The listing builds one solid part. Answer for the finished solid, in the listing's coordinates (mm). Give positions to 0.01 mm unless a question says otherwise; leave off trailing zeros. Order: outer loops, then holes, each group sorted by start corner. A loop starts at its lowest first (then second) coordinate and runs counter-clockwise, first axis right, second up.
Autodesk Inventor part; units mm, degrees
ref_plane "YZ Plane" through (0, 0, 0) normal (1, 0, 0) x (0, 1, 0)
ref_plane "XZ Plane" through (0, 0, 0) normal (0, 1, 0) x (-1, 0, 0)
ref_plane "XY Plane" through (0, 0, 0) normal (0, 0, 1) x (1, 0, 0)
sketch "Sketch1" plane through (0, 0, 0) normal (0, 0, 1) x (1, 0, 0)
  line L0 (0, 0) -> (1300, 0)
  line L1 (1300, 0) -> (1300, 50)
  line L2 (1300, 50) -> (0, 50)
  line L3 (0, 50) -> (0, 0)
  line L4 (0, 50) -> (50, 50)
  line L5 (50, 50) -> (50, 25)
  circle A0 centre (50, 25) radius 10.5
  line L6 (650, 50) -> (650, 17.5)
  circle A1 centre (1288, 40) radius 3
  circle A2 centre (1288, 10) radius 3
  line L7 (1182.5, 14.5) -> (1227.5, 14.5)
  line L8 (1227.5, 14.5) -> (1227.5, 35.5)
  line L9 (1227.5, 35.5) -> (1182.5, 35.5)
  line L10 (1182.5, 35.5) -> (1182.5, 14.5)
  dimension "d0" = 1300
  dimension "d1" = 50
  dimension "d4" = 50
  dimension "d5" = 21
  dimension "d10" = 6
  dimension "d11" = 6
  dimension "d14" = 45
  dimension "d17" = 21
  dimension "d18" = 14.5
  dimension "d19" = 25
  dimension "d20" = 12
  dimension "d21" = 12
  dimension "d22" = 10
extrude "Extrusion4" add sketch "Sketch1" along normal blind 6
equation "\"d18\" = -0.5 * d17 + 0.5 * d1"
properties part number "convyerwall"
1) Find section A-A (z = 2.25). Write down the section's boundary in (x, y).
Geometry says:
outline: (0, 0) - (1300, 0) - (1300, 50) - (0, 50) - close; hole circle Ø21 at (50, 25); hole (1182.5, 14.5) - (1227.5, 14.5) - (1227.5, 35.5) - (1182.5, 35.5) - close; hole circle Ø6 at (1288, 10); hole circle Ø6 at (1288, 40)
2) For a pull along X with two mould halves and no side action, classify faces 1 (the flat face through (641, 25, 6)), 2 (the cylindrical face through (39.51, 24.54, 2.96)) as +X half, -X half, draft (parallel to the pull), parting line (faces both ways), or undercut.
Geometry says:
face 1: draft
face 2: undercut
3) Find section C-C (x = 1209.5). Write down the section's boundary in (y, z), then the cut area to 3 significant figures.
Geometry says:
outline: (0, 0) - (14.5, 0) - (14.5, 6) - (0, 6) - close; (35.5, 0) - (50, 0) - (50, 6) - (35.5, 6) - close
area: 174 mm2
4) Straight lines are drawn through the part: probe 1 along Y at (x, z) = (1288, 2.45); probe 2 along X at (y, z) = (23.5, 2.55); probe 3 along X at (y, z) = (11, 2). For each, find the intervals that lie inside material, in ascending order.
Geometry says:
probe 1: y = 0 to 7, 13 to 37, 43 to 50
probe 2: x = 0 to 39.61, 60.39 to 1182.5, 1227.5 to 1300
probe 3: x = 0 to 1285.17, 1290.83 to 1300
5) Find section B-B (y = 25). Write down the section's boundary in (x, z), then the cut area to 3 significant figures.
Geometry says:
outline: (0, 0) - (39.5, 0) - (39.5, 6) - (0, 6) - close; (60.5, 0) - (1182.5, 0) - (1182.5, 6) - (60.5, 6) - close; (1227.5, 0) - (1300, 0) - (1300, 6) - (1227.5, 6) - close
area: 7,400 mm2
